For this review, take the finished solid that the model builds, in its own axes (mm). Face numbers are marked on the shaded views. Round coordinates to 2 decimals unless told otherwise and drop trailing zeros. Order: outer loops, then holes, each group sorted by start corner. A loop starts at its lowest first (then second) coordinate and runs counter-clockwise, first axis right, second up. Notation, with made-up numbers: M -35,6.5 L -12,6.5 A30 ccw -12,36.5 Z; hole C 82,-23 d8. An arc over 180 degrees is marked long. Answer as a JSON object with one key per item and string values.
Autodesk Inventor part; units mm, degrees
ref_plane "YZ Plane" through (0, 0, 0) normal (1, 0, 0) x (0, 1, 0)
ref_plane "XZ Plane" through (0, 0, 0) normal (0, 1, 0) x (-1, 0, 0)
ref_plane "XY Plane" through (0, 0, 0) normal (0, 0, 1) x (1, 0, 0)
sketch "Szkic1" plane through (0, 0, 0) normal (1, 0, 0) x (0, 1, 0)
  line L0 (9.9771, 19.755) -> (9.9771, -30.245) construction
  line L1 (5.4771, 19.755) -> (5.4771, -30.245)
  line L2 (14.4771, -30.245) -> (14.4771, 19.755)
  arc A0 (14.4771, 19.755) -> (5.4771, 19.755) centre (9.9771, 19.755) ccw
  arc A1 (5.4771, -30.245) -> (14.4771, -30.245) centre (9.9771, -30.245) ccw
  circle A2 centre (9.9771, 19.755) radius 1.75
  circle A3 centre (9.9771, -30.245) radius 1.75
  point P0 (0, 0)
  point P1 (9.9771, -5.245)
  dimension "d0" = 50
  dimension "d1" = 9
  dimension "d2" = 3.5
  dimension "d3" = 3.5
extrude "Wyciągnięcie proste1" add sketch "Szkic1" along normal blind 5
sketch "Szkic5" plane through (0, 0, 0) normal (-1, 0, 0) x (0, 0, 1)
  circle A0 centre (19.755, 9.9771) radius 1.75
  circle A1 centre (-30.245, 9.9771) radius 1.75
  circle A2 centre (19.755, 9.9771) radius 3
  circle A3 centre (-30.245, 9.9771) radius 3
  point P0 (0, 0)
  dimension "d20" = 6
  dimension "d21" = 6
extrude "Wyciągnięcie proste6" cut sketch "Szkic5" against normal blind 3 contours A0 | A1 | A2 | A3
properties part number "belka_2"
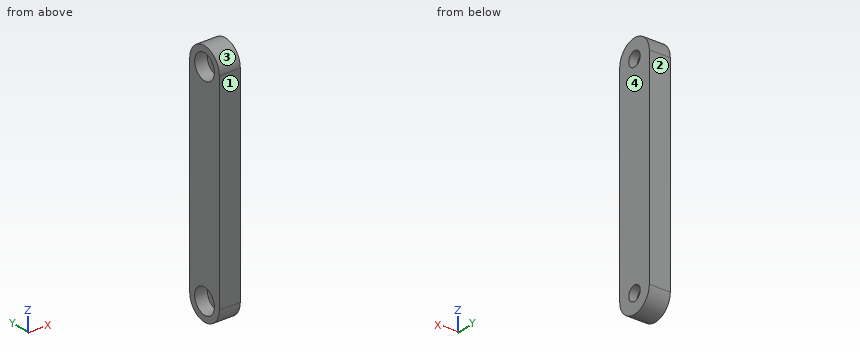
1) Add section A-A on y = 10.75. State the section outline as (x, z) points, and give its area (3 significant figures).
Geometry check:
{"outline": "M 0,-34.68 L 5,-34.68 L 5,-31.82 L 3,-31.82 L 3,-33.14 L 0,-33.14 Z; M 0,-27.35 L 3,-27.35 L 3,-28.67 L 5,-28.67 L 5,18.18 L 3,18.18 L 3,16.86 L 0,16.86 Z; M 0,22.65 L 3,22.65 L 3,21.33 L 5,21.33 L 5,24.19 L 0,24.19 Z", "area": "247 mm²"}
2) Add section C-C on z = -28. State the section outline as (x, y) points, and give its area (3 significant figures).
Geometry check:
{"outline": "M 0,5.48 L 5,5.48 L 5,14.48 L 0,14.48 L 0,11.97 L 3,11.97 L 3,7.99 L 0,7.99 Z", "area": "33.1 mm²"}
3) Add section D-D on x = 2.05. State the section outline as (y, z) points (3 decimals), and give its area (3 significant figures).
Geometry check:
{"outline": "M 5.477,-30.245 A4.5 ccw 14.477,-30.245 L 14.477,19.755 A4.5 ccw 5.477,19.755 Z; hole C 9.977,-30.245 d6; hole C 9.977,19.755 d6", "area": "457 mm²"}
4) For L1, parallel to Z at x = 2, y = 11; L2, parallel to Z at x = 2.45, y = 7.25; L3, parallel to Y at x = 2.25, z = -30, list the stretches that pass through material, from the lowest coordinate up.
Geometry check:
{"L1": "z = -34.63 to -33.07, -27.42 to 16.93, 22.58 to 24.14", "L2": "z = -33.82 to -31.5, -28.99 to 18.5, 21.01 to 23.33", "L3": "y = 5.48 to 6.99, 12.97 to 14.48"}
5) Add section B-B on x = 4.4. State the section outline as (y, z) points (3 decimals).
Geometry check:
{"outline": "M 5.477,-30.245 A4.5 ccw 14.477,-30.245 L 14.477,19.755 A4.5 ccw 5.477,19.755 Z; hole C 9.977,-30.245 d3.5; hole C 9.977,19.755 d3.5"}
6) Insertion check: P1, Ø1.8, axis at y = 11.5, z = -30.5, coming from the -X side; P2, Ø3, axis at x = 1.5, y = 8, coming from the +Z side. Each pin has a flat end and moves straight along its axis. Give the tip position at first contact, or say it passes through.
Geometry check:
{"P1": "stops at x = 3", "P2": "stops at z = 24.23"}
7) Mouldability with a two-part tool opening along Y and no side actions: class the marked faces 1, 2, 3 and 4 as +Y half, -Y half, draft (parallel to the pull), parting line (faces both ways), or undercut.
Geometry check:
{"face 1": "-Y half", "face 2": "+Y half", "face 3": "parting line", "face 4": "draft"}
